Solid Edge part; units mm, degrees
sketch "Sketch1" plane through (0, 0, 0) normal (0, 0, 1) x (1, 0, 0)
  line L0 (50, 140) -> (50, -140)
  line L1 (-20, -140) -> (50, -140)
  line L2 (-20, -130) -> (-20, -140)
  line L3 (20, -130) -> (-20, -130)
  line L4 (20, -110) -> (20, -130)
  line L5 (-20, -110) -> (20, -110)
  line L6 (-60, -80) -> (-20, -110)
  line L7 (-60, 80) -> (-60, -80)
  line L8 (-20, 110) -> (-60, 80)
  line L9 (20, 110) -> (-20, 110)
  line L10 (20, 130) -> (20, 110)
  line L11 (-20, 130) -> (20, 130)
  line L12 (-20, 140) -> (-20, 130)
  line L13 (50, 140) -> (-20, 140)
  dimension "D1" = 50
  dimension "D2" = 20
  dimension "D3" = 20
  dimension "D4" = 20
  dimension "D5" = 20
  dimension "D6" = 20
  dimension "D7" = 60
extrude "Protrusion1" add sketch "Sketch1" along normal blind 30
sketch "Sketch2" plane through (15, -140, 15) normal (0, -1, 0) x (1, 0, 0)
  circle A0 centre (-15, 0) radius 10
extrude "Cutout1" cut sketch "Sketch2" against normal up to next
mirror "Mirror1" about plane through (0, 0, 0) normal (0, -1, 0) of "Cutout1"
sketch "Sketch3" plane through (-5, 0, 30) normal (0, 0, 1) x (1, 0, 0)
  circle A0 centre (5, 0) radius 17.5
extrude "Cutout2" cut sketch "Sketch3" against normal up to next
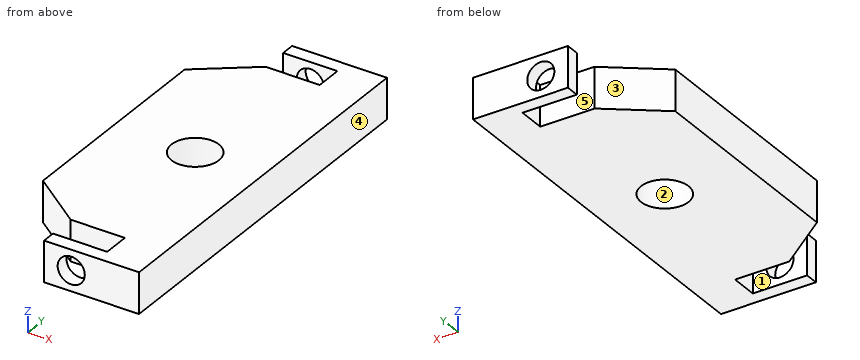
CAD build for the part. Positions are in the model's coordinates, mm. Face numbers are marked on the shaded views. A direction names the side the tool comes from. Round coordinates to 2 decimals unless told otherwise and drop trailing zeros. Order: outer loops, then holes, each group sorted by start corner. A loop starts at its lowest first (then second) coordinate and runs counter-clockwise, first axis right, second up. Notation, with made-up numbers: (56.25, 27) - (62.25, 27) arc R24 cw to (62.25, 55) - close; hole circle Ø2 at (58.25, 89.25). An arc over 180 degrees is marked (long way). Answer in a Markdown table with one row per item. Add a question column.
(1) Mould opens along X. For the marked faces 1, 2 and 3 say: +X half, -X half, draft (parallel to the pull), parting line (faces both ways), or undercut.
(2) Probe L1, parallel to Y at x = 0, z = 13.5; L2, parallel to Z at x = 0, y = 134.25; L3, parallel to Y at x = -16, z = 21.5. List the from-to ranges inside material, lowest first. Write a range as [from, to].
(3) 3-axis set-ups, long thin cutter, end or side, ignore diameter. For the marked faces 4 and 5: which of +Z, -Z, +X, -X, +Y, -Y reach the whole face in a straight line?
(4) Band-saw the part on C-C on x = 0. List the corners of the cut face in (y, z), and give its area (3 significant figures).
(5) Band-saw the part on B-B on y = 0. List the corners of the cut face in (x, z).
(6) Band-saw the part on A-A on z = 15. List the corners of the cut face in (x, y).
(7) Band-saw the part on D-D on x = -29. List the corners of the cut face in (y, z).
(8) Drop flat-ended pins along their axis: pin 1 Ø3 at (x, z) = (-23, 21.5) entering from -Y (3 decimals); pin 2 Ø10 at (x, z) = (-33, 19.5) entering from -Y; pin 3 Ø5 at (y, z) = (134, 14) entering from -X; pin 4 Ø21 at (x, y) = (0, 0) entering from -Z. Give the stop position or say it passes through.
Data:
| question | item | result |
|---|---|---|
| 1 | face 1 | draft |
| 1 | face 2 | undercut |
| 1 | face 3 | -X half |
| 2 | L1 | y = [-110, -17.5], [17.5, 110] |
| 2 | L2 | z = [0, 5], [25, 30] |
| 2 | L3 | y = [-140, -130], [-110, -7.09], [7.09, 110], [130, 140] |
| 3 | face 4 | +Z, -Z, +X, +Y, -Y |
| 3 | face 5 | +Z, -Z, -X |
| 4 | outline | (-140, 0) - (-130, 0) - (-130, 5) - (-140, 5) - close; (-140, 25) - (-130, 25) - (-130, 30) - (-140, 30) - close; (-110, 0) - (-17.5, 0) - (-17.5, 30) - (-110, 30) - close; (17.5, 0) - (110, 0) - (110, 30) - (17.5, 30) - close; (130, 0) - (140, 0) - (140, 5) - (130, 5) - close; (130, 25) - (140, 25) - (140, 30) - (130, 30) - close |
| 4 | area | 5,750 mm^2 |
| 5 | outline | (-60, 0) - (-17.5, 0) - (-17.5, 30) - (-60, 30) - close; (17.5, 0) - (50, 0) - (50, 30) - (17.5, 30) - close |
| 6 | outline | (-60, -80) - (-20, -110) - (20, -110) - (20, -130) - (10, -130) - (10, -140) - (50, -140) - (50, 140) - (10, 140) - (10, 130) - (20, 130) - (20, 110) - (-20, 110) - (-60, 80) - close; (-20, -140) - (-10, -140) - (-10, -130) - (-20, -130) - close; (-20, 130) - (-10, 130) - (-10, 140) - (-20, 140) - close; hole circle Ø35 at (0, 0) |
| 7 | outline | (-103.25, 0) - (103.25, 0) - (103.25, 30) - (-103.25, 30) - close |
| 8 | pin 1 | stops at y = -108.875 |
| 8 | pin 2 | stops at y = -104 |
| 8 | pin 3 | stops at x = -20 |
| 8 | pin 4 | passes through |
